from build123d import *

# Parameters (mm, degrees)
SKETCH1_W           = 70
SKETCH1_H           = 30
SKETCH1_R           = 4
SKETCH1_R_2         = 2.5
BOSS_EXTRUDE1_DEPTH = 4
SKETCH1_3_R         = 4
SKETCH1_3_R_2       = 2.5
BOSS_EXTRUDE2_DEPTH = 16.063
CHAMFER1_SIZE       = 5


with BuildPart() as part:
    # Sketch1 → Boss-Extrude1 (new body)
    with BuildSketch(Plane.XY):
        with Locations((15, 5)):
            Rectangle(SKETCH1_W, SKETCH1_H)
        with Locations((40, 0)):
            Circle(SKETCH1_R, mode=Mode.SUBTRACT)
        Circle(SKETCH1_R, mode=Mode.SUBTRACT)
        with Locations((40, 0)):
            Circle(SKETCH1_R)
        with Locations((40, 0)):
            Circle(SKETCH1_R_2, mode=Mode.SUBTRACT)
    extrude(amount=BOSS_EXTRUDE1_DEPTH)

    # Sketch1_3 → Boss-Extrude2 (add)
    with BuildSketch(Plane.XY):
        Circle(SKETCH1_3_R)
        Circle(SKETCH1_3_R_2, mode=Mode.SUBTRACT)
    extrude(amount=BOSS_EXTRUDE2_DEPTH)

    # Chamfer1
    chamfer1_edges = [part.edges().sort_by_distance(p)[0] for p in [
        (-4, 0, 4),
    ]]
    chamfer(chamfer1_edges, length=CHAMFER1_SIZE)


solid = part.part
Check sheet for the modelled part. Datum: model origin and axes. Units: mm. A direction names the side the tool comes from. Round coordinates to 2 decimals unless told otherwise and drop trailing zeros. Order: outer loops, then holes, each group sorted by start corner. A loop starts at its lowest first (then second) coordinate and runs counter-clockwise, first axis right, second up. Notation, with made-up numbers: M 15,-10.5 L 28,-10.5 A18 ccw 28,6.5 Z; hole C 7.5,48.25 d11. An arc over 180 degrees is marked long. One line per item, written item: value. Start each with the question number.
1. Section check B-B on y = 0. Enter the section's corners in (x, z).
2. Access from +Z, -Z, +X, -X, +Y, -Y to the whole of each face (thin tool, end or side, straight path). Record for faces 1 (the flat face through (50, 5, 2)), 2 (the cylindrical face through (-0.867, -3.905, 12.482)).
3. Scan lines: line 1 along Z through (x, y) = (15, 8.75); line 2 along Y through (x, z) = (40, 2.15); line 3 along Z through (x, y) = (-3, 6.25). Record each from-to range of solid material in increasing order.
4. Section check C-C on x = 0. Enter the section's corners in (y, z), and give its area (3 significant figures).
5. Release check for a two-part mould opening along X. For faces 3 (the cylindrical face through (42.31, -0.96, 1.97)), 4 (the flat face through (15, 20, 2)), 5 (the flat face through (-20, 5, 2)), 6 (the cylindrical face through (-0.54, -2.44, 7.92)) record: released by +X, released by -X, zero draft, split by the parting line, or undercut.
6. Section check D-D on z = 8. Enter the section's corners in (x, y), and give its area (3 significant figures).
7. Gauge pin test, flat ends, axial feed: P1, Ø4, axis at x = -1.5, y = 7.5, coming from the +Z side; P2, Ø3, axis at y = 7, z = 6, coming from the -X side; P3, Ø5, axis at y = 10, z = 8.5, coming from the +X side. Record the tip position at first contact, or that the pin passes through.
8. Section check A-A on x = 40. Enter the section's corners in (y, z), and give its area (3 significant figures).
Results found:
1. outline: M -20,0 L -2.5,0 L -2.5,16.06 L -4,16.06 L -4,9 L -9,4 L -20,4 Z; M 2.5,0 L 37.5,0 L 37.5,4 L 9,4 L 4,9 L 4,16.06 L 2.5,16.06 Z; M 42.5,0 L 50,0 L 50,4 L 42.5,4 Z
2. face 1: +Z, -Z, +X, +Y, -Y
2. face 2: +Z
3. line 1: 0 to 4
3. line 2: -10 to -2.5, 2.5 to 20
3. line 3: 0 to 6.07
4. outline: M -10,0 L -2.5,0 L -2.5,16.06 L -4,16.06 L -4,9 L -9,4 L -10,4 Z; M 2.5,0 L 20,0 L 20,4 L 9,4 L 4,9 L 4,16.06 L 2.5,16.06 Z
4. area: 161 mm^2
5. face 3: undercut
5. face 4: zero draft
5. face 5: released by -X
5. face 6: undercut
6. outline: C 0,0 d10; hole C 0,0 d5
6. area: 58.9 mm^2
7. P1: z = 7.35
7. P2: x = -5.48
7. P3: through
8. outline: M -10,0 L -2.5,0 L -2.5,4 L -10,4 Z; M 2.5,0 L 20,0 L 20,4 L 2.5,4 Z
8. area: 100 mm^2
